Verification items for this drawing (mm, ordinates from the low corner). Give positions to 0.01 mm unless a question says otherwise; leave off trailing zeros. Write each loop counter-clockwise with the first axis right and the second up, starting at its lowest first coordinate (ties: lowest second). Pieces come first, ordered by that corner, then holes. Notation, with made-up numbers: (87.25, 28) -> (118.25, 28) arc R30 cw to (118.25, 61) -> close; hole circle Ø8 at (83, 49.25). An arc over 180 degrees is marked (long way). Answer as a JSON object with one key per item and string values.
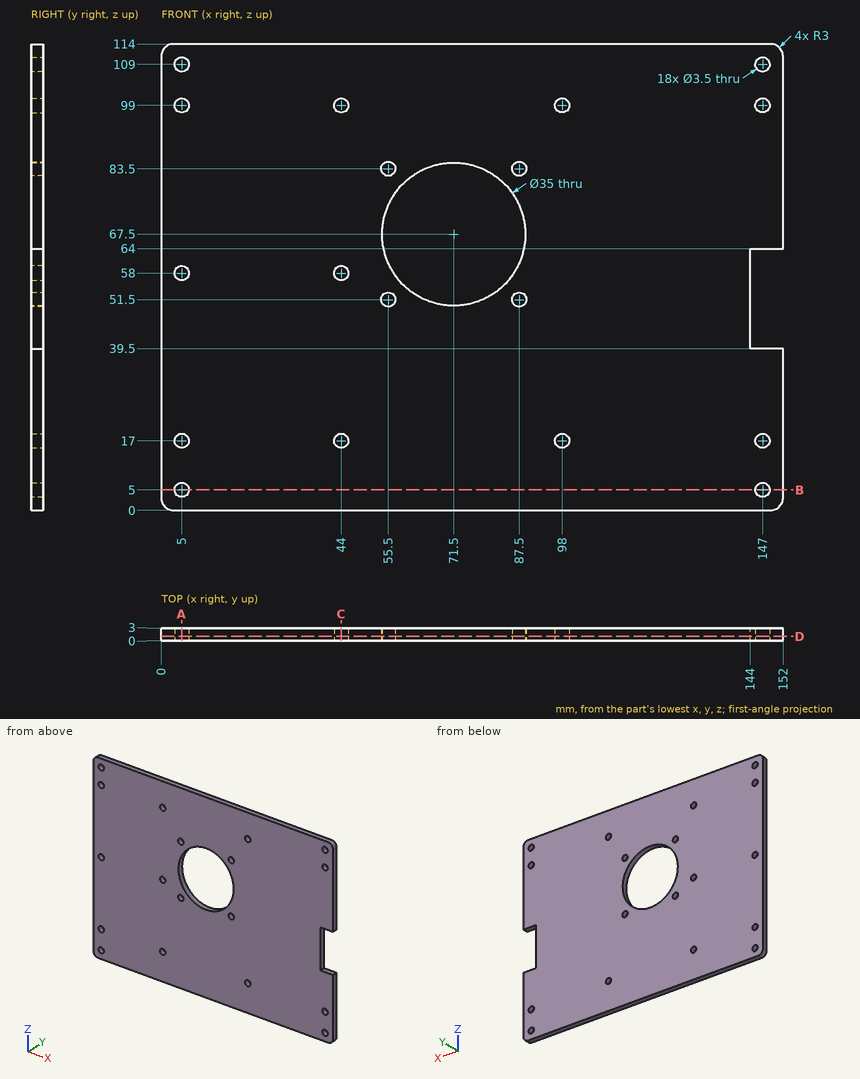
1. Sectioned sample at A-A, the plane x = 5. Enter the section's corners in (y, z), plus the area to 4 significant figures.
Determined:
{"outline": "(0, 0) -> (3, 0) -> (3, 3.25) -> (0, 3.25) -> close; (0, 6.75) -> (3, 6.75) -> (3, 15.25) -> (0, 15.25) -> close; (0, 18.75) -> (3, 18.75) -> (3, 56.25) -> (0, 56.25) -> close; (0, 59.75) -> (3, 59.75) -> (3, 97.25) -> (0, 97.25) -> close; (0, 100.75) -> (3, 100.75) -> (3, 107.25) -> (0, 107.25) -> close; (0, 110.75) -> (3, 110.75) -> (3, 114) -> (0, 114) -> close", "area": "289.5 mm^2"}
2. Sectioned sample at C-C, the plane x = 44. Enter the section's corners in (y, z), plus the area to 4 significant figures.
Determined:
{"outline": "(0, 0) -> (3, 0) -> (3, 15.25) -> (0, 15.25) -> close; (0, 18.75) -> (3, 18.75) -> (3, 56.25) -> (0, 56.25) -> close; (0, 59.75) -> (3, 59.75) -> (3, 97.25) -> (0, 97.25) -> close; (0, 100.75) -> (3, 100.75) -> (3, 114) -> (0, 114) -> close", "area": "310.5 mm^2"}
3. Sectioned sample at B-B, the plane z = 5. Enter the section's corners in (x, y), plus the area to 3 significant figures.
Determined:
{"outline": "(0, 0) -> (3.25, 0) -> (3.25, 3) -> (0, 3) -> close; (6.75, 0) -> (145.25, 0) -> (145.25, 3) -> (6.75, 3) -> close; (148.75, 0) -> (152, 0) -> (152, 3) -> (148.75, 3) -> close", "area": "435 mm^2"}
4. Go/stop test with flat-tipped pins: P1, Ø2, axis at x = 44, z = 58, coming from the +Y side; P2, Ø1.5, axis at y = 1.5, z = 56, coming from the +X side. Record where each tip stops, or that it passes through.
Determined:
{"P1": "through", "P2": "x = 144"}
5. Scan lines: L1, parallel to X at y = 1, z = 99; L2, parallel to Z at x = 5, y = 2; L3, parallel to Z at x = 147, y = 1.4. Record each from-to range of solid material in increasing order. Write a range as [from, to].
Determined:
{"L1": "[0, 3.25], [6.75, 42.25], [45.75, 96.25], [99.75, 145.25], [148.75, 152]", "L2": "[0, 3.25], [6.75, 15.25], [18.75, 56.25], [59.75, 97.25], [100.75, 107.25], [110.75, 114]", "L3": "[0, 3.25], [6.75, 15.25], [18.75, 39.5], [64, 97.25], [100.75, 107.25], [110.75, 114]"}
6. Sectioned sample at D-D, the plane y = 1.05. State how many separate pieces and enclosed holes the cut face has, plus the area to 3 significant figures.
Determined:
{"separate pieces": "1", "enclosed holes": "19", "area": "16,000 mm^2"}
